from build123d import *

# Parameters (mm, degrees)
BOSS_EXTRUDE1_DEPTH   = 10
FILLET1_R             = 5.08
F_5_0MM_DOWEL_HOLE1_D = 5
SKETCH14_R            = 2.5
CUT_EXTRUDE1_DEPTH    = 139.252681223
LPATTERN1_COUNT       = 5
LPATTERN1_PITCH       = 15


with BuildPart() as part:
    # Sketch1 → Boss-Extrude1 (new body)
    with BuildSketch(Plane.XY):
        Polygon((27.510468203, 50), (67.924987047, 120), (67.924987047, 81.9), (20.64, 0), (10, -99.432340815), (-10, -99.432340815), (-20.64, 0), (-67.924987047, 81.9), (-67.924987047, 120), (-27.510468203, 50), (-27.510468203, 100), (27.510468203, 100), align=None)
    extrude(amount=BOSS_EXTRUDE1_DEPTH)

    # Fillet1
    fillet1_edges = [part.edges().sort_by_distance(p)[0] for p in [
        (-27.510468203, 100, 5),
        (27.510468203, 100, 5),
        (27.510468203, 50, 5),
        (67.924987047, 81.9, 5),
        (20.64, 0, 5),
        (10, -99.432340815, 5),
        (-10, -99.432340815, 5),
        (-20.64, 0, 5),
        (-67.924987047, 81.9, 5),
        (-27.510468203, 50, 5),
    ]]
    fillet(fillet1_edges, radius=FILLET1_R)

    # Ø5.0mm Dowel Hole1 (through all)
    with Locations(Plane(origin=(0, 0, 0), x_dir=(-1, 0, 0), z_dir=(0, 0, -1))):
        with Locations((7.5, 25), (-7.5, 25)):
            f_5_0mm_dowel_hole1 = Hole(F_5_0MM_DOWEL_HOLE1_D / 2)

    # Sketch14 → Cut-Extrude1 (cut, through all)
    with BuildSketch(Plane.XY.offset(10)):
        with Locations((0, -89.432340815)):
            Circle(SKETCH14_R)
    extrude(amount=-CUT_EXTRUDE1_DEPTH, mode=Mode.SUBTRACT)

    # LPattern1: Ø5.0mm Dowel Hole1 ×5
    with Locations(*[(0, i * LPATTERN1_PITCH, 0) for i in range(1, LPATTERN1_COUNT)]):
        add(f_5_0mm_dowel_hole1, mode=Mode.SUBTRACT)


solid = part.part
Could you check a few things on this model? Use its own coordinates, in mm. A direction names the side the tool comes from. Give positions to 0.01 mm unless a question says otherwise; leave off trailing zeros. Order: outer loops, then holes, each group sorted by start corner. A loop starts at its lowest first (then second) coordinate and runs counter-clockwise, first axis right, second up.
1. For faces 4 (the cylindrical face through (6.96, 37.56, 5.07)), 5 (the flat face through (27.51, 82, 5)), which set-ups out of +Z, -Z, +X, -X, +Y, -Y let a thin tool reach every point of the face, with its end or its side?
2. Will these pins go through, and if not, where does the flat tip stop? P1, Ø3, axis at y = 78.5, z = 6.5, coming from the +X side; P2, Ø8, axis at x = -7.5, y = 85, coming from the -Z side; P3, Ø3, axis at x = -3.5, z = 4, coming from the +Y side; P4, Ø5, axis at y = 4, z = 6.5, coming from the -X side.
3. We'd pull the mould along Y, two halves only. Please class faces 1 (the flat face through (-5, 27, 10)), 2 (the cylindrical face through (-0.542, -91.873, 5.07)), 3 (the cylindrical face through (25.983, 98.551, 5.07)): pulls with the +Y half, pulls with the -Y half, needs draft (parallel to the pull), parting line crosses it, or undercut.
4. Suppose I cut it at C-C (z = 7.75). Give the number of separate pieces and of enclosed holes in the cut face, plus the area to 3 significant figures.
5. I need wall thicknesses on L1, parallel to Y at x = 0.5, z = 9.5; L2, parallel to X at y = 81, z = 3; L3, parallel to Y at x = -7.5, z = 6. Which ranges of each line are inside material? Lowest first, please.
6. Suppose I cut it at A-A (x = 0). List the corners of the cut face in (y, z) for me.
7. Suppose I cut it at B-B (y = 55). List the corners of the cut face in (x, z) for me, plus the area to 3 significant figures.
8. Suppose I cut it at D-D (y = 31). List the corners of the cut face in (x, z) for me.
Solved:
1. face 4: +Z, -Z
1. face 5: +Z, -Z, +Y
2. P1: stops at x = 66.83
2. P2: stops at z = 0
2. P3: stops at y = 100
2. P4: stops at x = -24.39
3. face 1: needs draft
3. face 2: undercut
3. face 3: pulls with the +Y half
4. separate pieces: 1
4. enclosed holes: 11
4. area: 11,400 mm2
5. L1: y = -99.43 to -91.88, -86.98 to 100
5. L2: x = -67.39 to -45.41, -27.51 to 27.51, 45.41 to 67.39
5. L3: y = -98.99 to 22.5, 27.5 to 37.5, 42.5 to 52.5, 57.5 to 67.5, 72.5 to 82.5, 87.5 to 100
6. outline: (-99.43, 0) - (-91.93, 0) - (-91.93, 10) - (-99.43, 10) - close; (-86.93, 0) - (100, 0) - (100, 10) - (-86.93, 10) - close
7. outline: (-52.39, 0) - (-10, 0) - (-10, 10) - (-52.39, 10) - close; (-5, 0) - (5, 0) - (5, 10) - (-5, 10) - close; (10, 0) - (52.39, 0) - (52.39, 10) - (10, 10) - close
7. area: 948 mm2
8. outline: (-38.54, 0) - (38.54, 0) - (38.54, 10) - (-38.54, 10) - close
